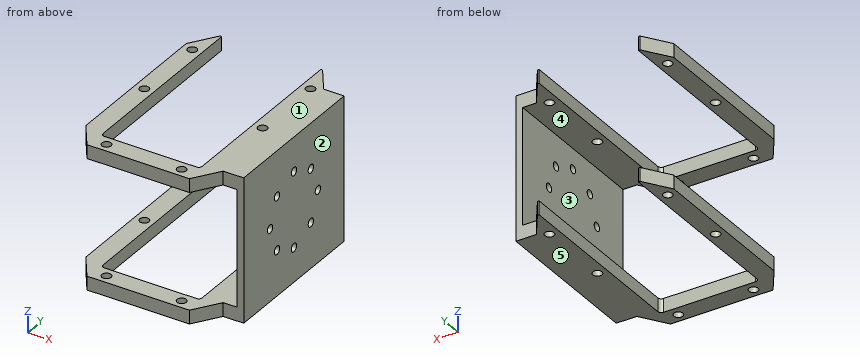
```python
from build123d import *

# Parameters (mm, degrees)
EXTRUDE_2_DEPTH     = 42
SKETCH_2_R          = 1.35
CUT_EXTRUDE_1_DEPTH = 45
CUT_EXTRUDE_2_DEPTH = 45
SKETCH_4_W          = 4
SKETCH_4_H          = 46.1
EXTRUDE_3_DEPTH     = 4
SKETCH_5_W          = 2
SKETCH_5_H          = 46.1
EXTRUDE_4_DEPTH     = 42
SKETCH_6_R          = 1.225
CUT_EXTRUDE_3_DEPTH = 10


with BuildPart() as part:
    # Sketch 1 → Extrude 2 (new body)
    with BuildSketch(Plane.XY):
        with BuildLine():
            Line((-14.5, -41.5), (-14.5, 11.5))
            Line((-14.5, 11.5), (-14.5, 13))
            Line((-14.5, 13), (-15, 13))
            Line((-15, 13), (-20.1, 5.5))
            Line((-20.1, 5.5), (-20.1, -40.6))
            Line((-20.1, -40.6), (-15, -48.1))
            Line((-15, -48.1), (15, -48.1))
            Line((15, -48.1), (20.1, -40.6))
            Line((20.1, -40.6), (20.1, 5.5))
            Line((20.1, 5.5), (15, 13))
            Line((15, 13), (14.5, 13))
            Line((14.5, 13), (14.5, 11.5))
            Line((14.5, 11.5), (14.5, -41.5))
            ThreePointArc((14.5, -41.5), (14.207106781, -42.207106781), (13.5, -42.5))
            Line((13.5, -42.5), (-13.5, -42.5))
            ThreePointArc((-13.5, -42.5), (-14.207106781, -42.207106781), (-14.5, -41.5))
        make_face()
    extrude(amount=EXTRUDE_2_DEPTH)

    # Sketch 2 → Cut-Extrude 1 (cut)
    with BuildSketch(Plane(origin=(0, 0, 0), x_dir=(-1, 0, 0), z_dir=(0, 0, -1))):
        with Locations((-11, -45.405560676)):
            Circle(SKETCH_2_R)
        with Locations((11, -45.405560676)):
            Circle(SKETCH_2_R)
        with Locations((17.3, 3.87)):
            Circle(SKETCH_2_R)
        with Locations((17.3, -18.13)):
            Circle(SKETCH_2_R)
        with Locations((-17.3, 3.87)):
            Circle(SKETCH_2_R)
        with Locations((-17.3, -18.13)):
            Circle(SKETCH_2_R)
    extrude(amount=-CUT_EXTRUDE_1_DEPTH, mode=Mode.SUBTRACT)

    # Sketch 3 → Cut-Extrude 2 (cut)
    with BuildSketch(Plane(origin=(20.1, 0, 0), x_dir=(0, 0, -1), z_dir=(1, 0, 0))):
        Polygon((-38, 5.5), (-38, -40.6), (-38, -48.1), (-4, -48.1), (-4, -40.6), (-4, 5.5), (-4, 13), (-38, 13), align=None)
    extrude(amount=-CUT_EXTRUDE_2_DEPTH, mode=Mode.SUBTRACT)


with BuildPart() as cut_extrude_2_piece_1:
    # of the separate pieces the step leaves, piece 1, a body of its own (cut_extrude_2_pieces)
    add(part.part.solids().sort_by_distance((-14.5, -41.5, 38))[0])



with BuildPart() as cut_extrude_2_piece_2:
    # of the separate pieces the step leaves, piece 2, a body of its own (cut_extrude_2_pieces)
    add(part.part.solids().sort_by_distance((-14.5, -41.5, 0))[0])


with BuildPart() as cut_extrude_2_piece_1_1:
    add(cut_extrude_2_piece_1.part)

    add(cut_extrude_2_piece_2.part)  # Extrude 3 merges Cut-Extrude 2 piece 2
    # Sketch 4 → Extrude 3 (add)
    with BuildSketch(Plane(origin=(20.1, 0, 0), x_dir=(0, 0, -1), z_dir=(1, 0, 0))):
        with Locations((-40, -17.55)):
            Rectangle(SKETCH_4_W, SKETCH_4_H)
        with Locations((-2, -17.55)):
            Rectangle(SKETCH_4_W, SKETCH_4_H)
    extrude(amount=EXTRUDE_3_DEPTH)

    # Sketch 5 → Extrude 4 (add)
    with BuildSketch(Plane.XY.offset(42)):
        with Locations((25.1, -17.55)):
            Rectangle(SKETCH_5_W, SKETCH_5_H)
    extrude(amount=-EXTRUDE_4_DEPTH)

    # Sketch 6 → Cut-Extrude 3 (cut)
    with BuildSketch(Plane(origin=(26.1, 0, 0), x_dir=(0, 0, -1), z_dir=(1, 0, 0))):
        with Locations((-28.801064549, -9.782397482)):
            Circle(SKETCH_6_R)
        with Locations((-21.022889956, -6.560572075)):
            Circle(SKETCH_6_R)
        with Locations((-13.244715363, -9.782397482)):
            Circle(SKETCH_6_R)
        with Locations((-10.022889956, -17.560572075)):
            Circle(SKETCH_6_R)
        with Locations((-13.244715363, -25.338746668)):
            Circle(SKETCH_6_R)
        with Locations((-21.022889956, -28.560572075)):
            Circle(SKETCH_6_R)
        with Locations((-28.801064549, -25.338746668)):
            Circle(SKETCH_6_R)
        with Locations((-32.022889956, -17.560572075)):
            Circle(SKETCH_6_R)
    extrude(amount=-CUT_EXTRUDE_3_DEPTH, mode=Mode.SUBTRACT)


solid = cut_extrude_2_piece_1_1.part
```
Geometry: final body of the model. Coordinates: model frame, mm. Face numbers are marked on the shaded views. A direction names the side the tool comes from. Coordinates: 2 decimals unless noted, no trailing zeros. Write each loop counter-clockwise with the first axis right and the second up, starting at its lowest first coordinate (ties: lowest second). Pieces come first, ordered by that corner, then holes. Notation, with made-up numbers: M 44.25,55 L 67.25,55 A15 cw 67.25,59 Z; hole C -5,76.25 d2. An arc over 180 degrees is marked long. Use CSV: the item, a comma, the result in double quotes. Start each with the question number.
1. Cut plane B-B on y = -31. Return the cut outline in (x, z), plus the area to 3 significant figures.
2. Reachability of the marked faces 4 and 5 from +Z, -Z, +X, -X, +Y, -Y: full face, straight path, thin tool, end or side. Return the list, or none.
3. First-contact query: P1, Ø1, axis at y = -2.5, z = 21.5, coming from the -X side; P2, Ø5, axis at x = 23.5, z = 25, coming from the +Y side; P3, Ø3, axis at x = 12, z = 5, coming from the +Y side. Flat tips, straight axial feed; report the tip coordinate or a pass-through.
4. Mould query, pull axis Z, two halves, no side actions, for the marked faces 1, 2 and 3. Classes: pulls with the +Z half, pulls with the -Z half, needs draft (parallel to the pull), parting line crosses it, or undercut.
5. Ray query, probe 1 along Z at (x, y) = (20, -39.5); probe 2 along Y at (x, z) = (-17.3, 1.3); probe 3 along X at (y, z) = (-18, 6). Return the intervals inside material, ascending.
6. Cut plane C-C on x = -11. Return the cut outline in (y, z).
7. Cut plane D-D on x = 21.5. Return the cut outline in (y, z), plus the area to 3 significant figures.
8. Cut plane A-A on x = 0. Return the cut outline in (y, z), plus the area to 3 significant figures.
Entries:
1,outline,"M -20.1,0 L -14.5,0 L -14.5,4 L -20.1,4 Z; M -20.1,38 L -14.5,38 L -14.5,42 L -20.1,42 Z; M 14.5,0 L 26.1,0 L 26.1,42 L 14.5,42 L 14.5,38 L 24.1,38 L 24.1,4 L 14.5,4 Z"
1,area,"206 mm²"
2,face 4,"-X, +Y, -Y"
2,face 5,"-Z, +X, -X, +Y, -Y"
3,P1,"x = 24.1"
3,P2,"y = 5.5"
3,P3,"y = -42.5"
4,face 1,"pulls with the +Z half"
4,face 2,"needs draft"
4,face 3,"undercut"
5,probe 1,"0 to 4, 38 to 42"
5,probe 2,"-44.72 to -19.48, -16.78 to 2.52, 5.22 to 9.62"
5,probe 3,"24.1 to 26.1"
6,outline,"M -48.1,0 L -46.76,0 L -46.76,4 L -48.1,4 Z; M -48.1,38 L -46.76,38 L -46.76,42 L -48.1,42 Z; M -44.06,0 L -42.5,0 L -42.5,4 L -44.06,4 Z; M -44.06,38 L -42.5,38 L -42.5,42 L -44.06,42 Z"
7,outline,"M -40.6,0 L 5.5,0 L 5.5,4 L -40.6,4 Z; M -40.6,38 L 5.5,38 L 5.5,42 L -40.6,42 Z"
7,area,"369 mm²"
8,outline,"M -48.1,0 L -42.5,0 L -42.5,4 L -48.1,4 Z; M -48.1,38 L -42.5,38 L -42.5,42 L -48.1,42 Z"
8,area,"44.8 mm²"
